from build123d import *

# Parameters (mm, degrees)
F1_DEPTH = 7
F3_DEPTH = 7


with BuildPart() as f1:
    # F0 (on Top) → F1 (new body)
    with BuildSketch(Plane.XY):
        with BuildLine():
            Line((-13.8564064606, 8), (-10.6000951209, 13.6400966855))
            ThreePointArc((-10.6000951209, 13.6400966855), (-11.4165365305, 14.7949535985), (-12.1076766085, 16.0288889524))
            Line((-12.1076766085, 16.0288889524), (-19.9352633315, 2.4711110476))
            ThreePointArc((-19.9352633315, 2.4711110476), (-18.5210739294, 2.4895338594), (-17.1127178002, 2.3599033145))
            Line((-17.1127178002, 2.3599033145), (-13.8564064606, 8))
        make_face()
        with BuildLine():
            Line((-7.8262379212, 11), (-4.8262379212, 11))
            Line((-4.8262379212, 11), (-4.8262379212, 12.1152932503))
            ThreePointArc((-4.8262379212, 12.1152932503), (0, 33), (4.8262379212, 12.1152932503))
            Line((4.8262379212, 12.1152932503), (4.8262379212, 11))
            Line((4.8262379212, 11), (7.8262379212, 11))
            ThreePointArc((7.8262379212, 11), (9.3072533528, 12.2211946012), (10.6000951209, 13.6400966855))
            ThreePointArc((10.6000951209, 13.6400966855), (11.4165365305, 14.7949535985), (12.1076766085, 16.0288889524))
            ThreePointArc((12.1076766085, 16.0288889524), (0, 35.5), (-12.1076766085, 16.0288889524))
            ThreePointArc((-12.1076766085, 16.0288889524), (-11.4165365305, 14.7949535985), (-10.6000951209, 13.6400966855))
            ThreePointArc((-10.6000951209, 13.6400966855), (-9.3072533528, 12.2211946012), (-7.8262379212, 11))
        make_face()
        with BuildLine():
            ThreePointArc((12.1076766085, 16.0288889524), (11.4165365305, 14.7949535985), (10.6000951209, 13.6400966855))
            Line((10.6000951209, 13.6400966855), (13.8564064606, 8))
            Line((13.8564064606, 8), (17.1127178002, 2.3599033145))
            ThreePointArc((17.1127178002, 2.3599033145), (18.5210739294, 2.4895338594), (19.9352633315, 2.4711110476))
            Line((19.9352633315, 2.4711110476), (12.1076766085, 16.0288889524))
        make_face()
        with BuildLine():
            ThreePointArc((0, -11), (-3.2138778591, -10.5200279993), (-6.1472881936, -9.1219980194))
            Line((-6.1472881936, -9.1219980194), (-8.0790327684, -10.2372912697))
            ThreePointArc((-8.0790327684, -10.2372912697), (-28.5788383249, -16.5), (-12.9052706897, -1.8780019806))
            Line((-12.9052706897, -1.8780019806), (-10.9735261148, -0.7627087303))
            ThreePointArc((-10.9735261148, -0.7627087303), (-9.5262794416, 5.5), (-4.8262379212, 9.8847067497))
            Line((-4.8262379212, 9.8847067497), (-4.8262379212, 11))
            Line((-4.8262379212, 11), (-7.8262379212, 11))
            ThreePointArc((-7.8262379212, 11), (-11.6913429511, 6.75), (-13.4393984023, 1.2777208559))
            ThreePointArc((-13.4393984023, 1.2777208559), (-15.2374916656, 1.9497205423), (-17.1127178002, 2.3599033145))
            ThreePointArc((-17.1127178002, 2.3599033145), (-18.5210739294, 2.4895338594), (-19.9352633315, 2.4711110476))
            ThreePointArc((-19.9352633315, 2.4711110476), (-30.7439018343, -17.75), (-7.8275867229, -18.5))
            Line((-7.8275867229, -18.5), (7.8275867229, -18.5))
            ThreePointArc((7.8275867229, -18.5), (30.7439018343, -17.75), (19.9352633315, 2.4711110476))
            ThreePointArc((19.9352633315, 2.4711110476), (18.5210739294, 2.4895338594), (17.1127178002, 2.3599033145))
            ThreePointArc((17.1127178002, 2.3599033145), (15.2374916656, 1.9497205423), (13.4393984023, 1.2777208559))
            ThreePointArc((13.4393984023, 1.2777208559), (11.6913429511, 6.75), (7.8262379212, 11))
            Line((7.8262379212, 11), (4.8262379212, 11))
            Line((4.8262379212, 11), (4.8262379212, 9.8847067497))
            ThreePointArc((4.8262379212, 9.8847067497), (9.5262794416, 5.5), (10.9735261148, -0.7627087303))
            Line((10.9735261148, -0.7627087303), (12.9052706897, -1.8780019806))
            ThreePointArc((12.9052706897, -1.8780019806), (28.5788383249, -16.5), (8.0790327684, -10.2372912697))
            Line((8.0790327684, -10.2372912697), (6.1472881936, -9.1219980194))
            ThreePointArc((6.1472881936, -9.1219980194), (3.2138778591, -10.5200279993), (0, -11))
        make_face()
        with BuildLine():
            ThreePointArc((-5.613160481, -12.2777208559), (-2.8723482071, -13.1908913943), (0, -13.5))
            ThreePointArc((0, -13.5), (2.8723482071, -13.1908913943), (5.613160481, -12.2777208559))
            ThreePointArc((5.613160481, -12.2777208559), (5.9302383129, -14.1709151435), (6.5126226793, -16))
            Line((6.5126226793, -16), (0, -16))
            Line((0, -16), (-6.5126226793, -16))
            ThreePointArc((-6.5126226793, -16), (-5.9302383129, -14.1709151435), (-5.613160481, -12.2777208559))
        make_face(mode=Mode.SUBTRACT)
    extrude(amount=F1_DEPTH)

    # F2 (on face) → F3 (join)
    with BuildSketch(Plane.XY.offset(7)):
        with BuildLine():
            ThreePointArc((12.8426779045, 26.1612046623), (13.8763872298, 28.9318631067), (15.9538742155, 31.0364179313))
            ThreePointArc((15.9538742155, 31.0364179313), (8.3843737037, 34.7244815518), (0, 35.5))
            ThreePointArc((0, 35.5), (7.9395760926, 32.9184766094), (12.8426779045, 26.1612046623))
        make_face()
        with BuildLine():
            ThreePointArc((-30.7439018343, -17.75), (-32.4780250439, -9.5833637133), (-29.0776067834, -1.9585170132))
            ThreePointArc((-29.0776067834, -1.9585170132), (-31.9939220442, -2.4486276996), (-34.8552634787, -1.7017486063))
            ThreePointArc((-34.8552634787, -1.7017486063), (-34.264470009, -10.1011601537), (-30.7439018343, -17.75))
        make_face()
        with BuildLine():
            ThreePointArc((18.9013892633, -29.334669325), (25.8800963053, -24.6233213981), (30.7439018343, -17.75))
            ThreePointArc((30.7439018343, -17.75), (24.5384489513, -23.3351128962), (16.2349288789, -24.202687649))
            ThreePointArc((16.2349288789, -24.2026876491), (18.1175348143, -26.4832354072), (18.9013892633, -29.334669325))
        make_face()
    extrude(amount=-F3_DEPTH)


solid = f1.part
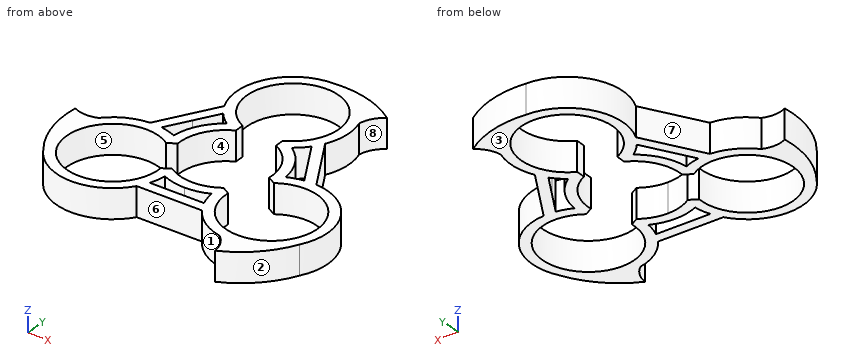
Design review of the part built by this model. Coordinates are the model's own, in mm. Face numbers are marked on the shaded views. A direction names the side the tool comes from. Coordinates: 2 decimals unless noted, no trailing zeros. Order: outer loops, then holes, each group sorted by start corner. A loop starts at its lowest first (then second) coordinate and runs counter-clockwise, first axis right, second up. Notation, with made-up numbers: (6.5, 18.5) -> (13.5, 18.5) arc R35 ccw to (13.5, 53.5) -> close; hole circle Ø8 at (-32.75, 86.25). An arc over 180 degrees is marked (long way). Use one line per item in the form item = value. Start each with the question number.
(1) Insertion check: pin 1 (1.5 mm diameter, centred on y = -20, z = 5, fed in from +X); pin 2 (3.5 mm diameter, centred on x = 0.5, z = 3.5, fed in from +Y); pin 3 (3 mm diameter, centred on y = -9, z = 2.5, fed in from -X); pin 4 (1 mm diameter, centred on x = -2.5, z = 5, fed in from -Y). Each pin has a flat end and moves straight along its axis. Give the tip position at first contact, or say it passes through.
(2) For probe 1 along X at (y, z) = (22, 3); probe 2 along Y at (x, z) = (2, 6.75); probe 3 along Y at (x, z) = (-7.5, 5.5), list the stretches that pass through material, from the lowest coordinate up.
(3) Add section C-C on y = -20. State the section outline as (x, z) points.
(4) For the marked faces 5, 6, 7 and 8, list the 3-axis set-ups (+Z, -Z, +X, -X, +Y, -Y) from which the entire face can be reached by the end or side of a thin tool; tool diameter is ignored.
(5) The part is to be moulded in two halves that separate along X. For the marked faces 1, 2, 3 and 4, say which applies: +X half, -X half, draft (parallel to the pull), parting line (faces both ways), or undercut.
(6) Add section B-B on x = 21. State the section outline as (y, z) points.
(7) Add section D-D on z = 5.25. Give the number of separate pieces and of enclosed holes in the cut face, plus the area to 3 significant figures.
(8) Add section A-A on y = 22. State the section outline as (x, z) points, plus the area to 3 significant figures.
Answer block:
q1.pin_1 = 29.98
q1.pin_2 = 35.59
q1.pin_3 = -34.78
q1.pin_4 = -18.5
q2.probe_1 = -13.5 to -11, 11 to 13.5
q2.probe_2 = -18.5 to -16, -13.35 to -10.82, 32.82 to 35.59
q2.probe_3 = -18.5 to -9.9, 8.05 to 13.95, 30.05 to 33.22
q3.outline = (-29.11, 0) -> (-25.38, 0) -> (-25.38, 7) -> (-29.11, 7) -> close; (-12.73, 0) -> (-8.99, 0) -> (-8.99, 7) -> (-12.73, 7) -> close; (8.99, 0) -> (12.73, 0) -> (12.73, 7) -> (8.99, 7) -> close; (25.38, 0) -> (29.54, 0) -> (29.54, 7) -> (25.38, 7) -> close
q4.face_5 = +Z, -Z
q4.face_6 = +Z, -Z, -Y
q4.face_7 = +Z, -Z, -X
q4.face_8 = +Z, -Z, +X
q5.face_1 = undercut
q5.face_2 = +X half
q5.face_3 = draft
q5.face_4 = undercut
q6.outline = (-28.29, 0) -> (-21.83, 0) -> (-21.83, 7) -> (-28.29, 7) -> close; (-0.17, 0) -> (2.36, 0) -> (2.36, 7) -> (-0.17, 7) -> close
q7.separate_pieces = 1
q7.enclosed_holes = 4
q7.area = 793 mm²
q8.outline = (-13.5, 0) -> (-11, 0) -> (-11, 7) -> (-13.5, 7) -> close; (11, 0) -> (13.5, 0) -> (13.5, 7) -> (11, 7) -> close
q8.area = 35.0 mm²
